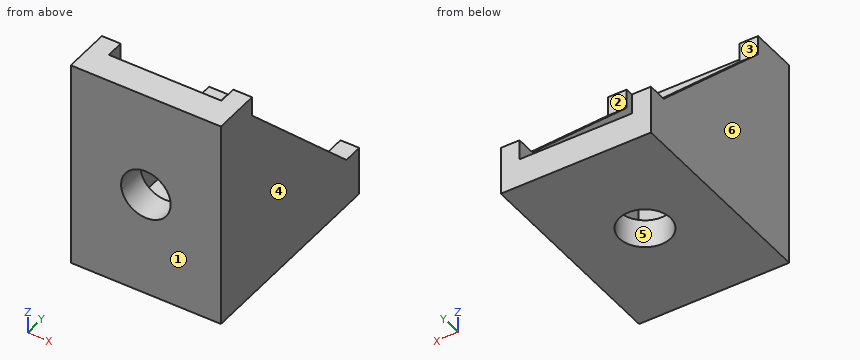
```python
from build123d import *

# Parameters (mm, degrees)
SKETCH1_W           = 20
SKETCH1_H           = 28
SKETCH1_R           = 3.4
BOSS_EXTRUDE1_DEPTH = 3.8
SKETCH2_W           = 20
SKETCH2_H           = 28
SKETCH2_R           = 3.3
BOSS_EXTRUDE2_DEPTH = 3.9
SKETCH3_W           = 6.5
SKETCH3_H           = 24.1
BOSS_EXTRUDE3_DEPTH = 2.5
SKETCH4_W           = 28
SKETCH4_H           = 6.3
BOSS_EXTRUDE4_DEPTH = 2.5
BOSS_EXTRUDE5_DEPTH = 2.5


with BuildPart() as part:
    # Sketch1 → Boss-Extrude1 (new body)
    with BuildSketch(Plane.XY):
        Rectangle(SKETCH1_W, SKETCH1_H)
        Circle(SKETCH1_R, mode=Mode.SUBTRACT)
    extrude(amount=BOSS_EXTRUDE1_DEPTH)

    # Sketch2 → Boss-Extrude2 (add)
    with BuildSketch(Plane.XZ.offset(14)):
        with Locations((0, 14)):
            Rectangle(SKETCH2_W, SKETCH2_H)
        with Locations((0, 14)):
            Circle(SKETCH2_R, mode=Mode.SUBTRACT)
    extrude(amount=-BOSS_EXTRUDE2_DEPTH)

    # Sketch3 → Boss-Extrude3 (add)
    with BuildSketch(Plane.ZY.offset(10)):
        with Locations((3.25, 1.95)):
            Rectangle(SKETCH3_W, SKETCH3_H)
    boss_extrude3 = extrude(amount=-BOSS_EXTRUDE3_DEPTH)

    # Mirror1: Boss-Extrude3 across plane
    add(boss_extrude3.mirror(Plane(origin=(0, 0, 0), x_dir=(0, 0, 1), z_dir=(1, 0, 0))))

    # Sketch4 → Boss-Extrude4 (add)
    with BuildSketch(Plane.ZY.offset(10)):
        with Locations((14, -10.85)):
            Rectangle(SKETCH4_W, SKETCH4_H)
    boss_extrude4 = extrude(amount=-BOSS_EXTRUDE4_DEPTH)

    # Mirror2: Boss-Extrude4 across plane
    add(boss_extrude4.mirror(Plane(origin=(0, 0, 0), x_dir=(0, 0, 1), z_dir=(1, 0, 0))))

    # Sketch5 → Boss-Extrude5 (add)
    with BuildSketch(Plane.ZY.offset(10)):
        Polygon((6.5, 11.4), (25.4, -7.7), (6.5, -7.7), align=None)
    boss_extrude5 = extrude(amount=-BOSS_EXTRUDE5_DEPTH)

    # Mirror3: Boss-Extrude5 across plane
    add(boss_extrude5.mirror(Plane(origin=(0, 0, 0), x_dir=(0, 0, 1), z_dir=(1, 0, 0))))


solid = part.part
```
Input: part model. Units: mm. Frame: model coordinates. Face numbers are marked on the shaded views. A direction names the side the tool comes from. Coordinates: 2 decimals unless noted, no trailing zeros. Order: outer loops, then holes, each group sorted by start corner. A loop starts at its lowest first (then second) coordinate and runs counter-clockwise, first axis right, second up. Notation, with made-up numbers: (73, 30.5) - (125, 30.5) arc R20 ccw to (125, 45.5) - close; hole circle Ø5 at (32, -27). An arc over 180 degrees is marked (long way). Return JSON: item names as keys, results as strings.
Q1. Access query for the marked faces 1 and 2. Directions: +Z, -Z, +X, -X, +Y, -Y. A direction counts if a zero-diameter tool reaches every point of the face in a straight line with its end or side. Return the directions, or none.
The answers:
{"face 1": "+Z, -Z, +X, -X, -Y", "face 2": "+Z, +X, -X, +Y"}
Q2. Ray query, probe 1 along Z at (x, y) = (0, -11.9); probe 2 along Y at (x, z) = (0, 1); probe 3 along X at (y, z) = (-6.75, 4.75). Return the intervals inside material, ascending.
The answers:
{"probe 1": "z = 0 to 10.7, 17.3 to 28", "probe 2": "y = -14 to -3.4, 3.4 to 14", "probe 3": "x = -10 to -7.5, 7.5 to 10"}
Q3. First-contact query: pin 1 (1.5 mm diameter, centred on x = -1.5, y = -11, fed in from -Z); pin 2 (7.5 mm diameter, centred on x = -2, y = 3, fed in from +Z); pin 3 (0.8 mm diameter, centred on x = -8.5, z = 26, fed in from +Y); pin 4 (4.5 mm diameter, centred on x = 1, z = 20.5, fed in from +Y). Flat tips, straight axial feed; report the tip coordinate or a pass-through.
The answers:
{"pin 1": "stops at z = 0", "pin 2": "stops at z = 3.8", "pin 3": "stops at y = -7.7", "pin 4": "stops at y = -10.1"}
Q4. Cut plane A-A (x = 0). Return loops of the section in (y, z), then the cut area to 3 significant figures.
The answers:
{"outline": "(-14, 0) - (-3.4, 0) - (-3.4, 3.8) - (-10.1, 3.8) - (-10.1, 10.7) - (-14, 10.7) - close; (-14, 17.3) - (-10.1, 17.3) - (-10.1, 28) - (-14, 28) - close; (3.4, 0) - (14, 0) - (14, 3.8) - (3.4, 3.8) - close", "area": "149 mm2"}
Q5. Draft query along X for the marked faces 3, 4, 5 and 6. Return one class per face: +X half, -X half, draft (parallel to the pull), parting line (faces both ways), or undercut.
The answers:
{"face 3": "draft", "face 4": "+X half", "face 5": "undercut", "face 6": "-X half"}
Q6. Cut plane C-C (z = 14). Return loops of the section in (x, y).
The answers:
{"outline": "(-10, -14) - (-3.3, -14) - (-3.3, -10.1) - (-7.5, -10.1) - (-7.5, 3.82) - (-10, 3.82) - close; (3.3, -14) - (10, -14) - (10, 3.82) - (7.5, 3.82) - (7.5, -10.1) - (3.3, -10.1) - close"}
Q7. Cut plane D-D (x = -6). Return loops of the section in (y, z).
The answers:
{"outline": "(-14, 0) - (14, 0) - (14, 3.8) - (-10.1, 3.8) - (-10.1, 28) - (-14, 28) - close"}
Q8. Cut plane B-B (y = 0). Return loops of the section in (x, z), then the cut area to 3 significant figures.
The answers:
{"outline": "(-10, 0) - (-3.4, 0) - (-3.4, 3.8) - (-7.5, 3.8) - (-7.5, 17.78) - (-10, 17.78) - close; (3.4, 0) - (10, 0) - (10, 17.78) - (7.5, 17.78) - (7.5, 3.8) - (3.4, 3.8) - close", "area": "120 mm2"}
